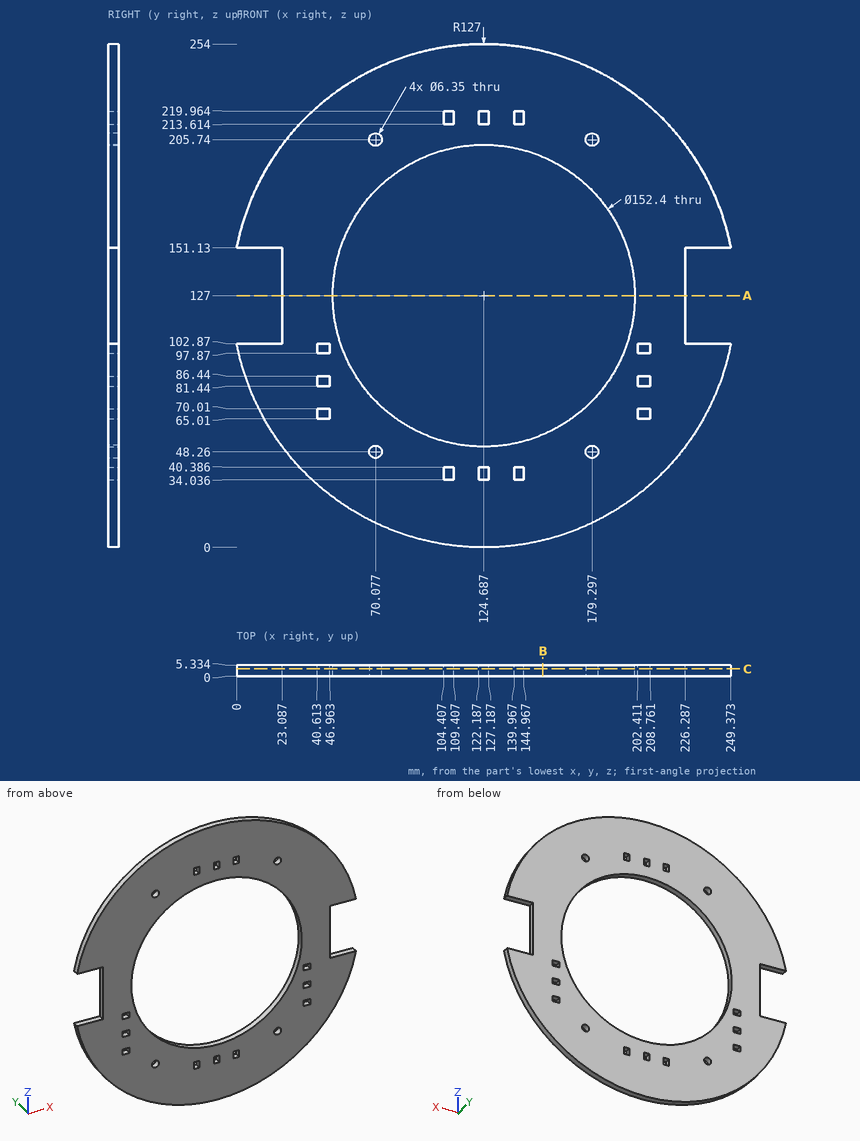
Here's the drawing with two shaded views (mm, measured from the low corner). I have some questions. Give positions to 0.01 mm unless a question says otherwise; leave off trailing zeros. Loops run counter-clockwise (first coordinate to the right, second up) from the corner with the lowest first, then second, coordinate; pieces in that order, holes last. Notation, with made-up numbers: (-24.5, 80.25) - (32.5, 80.25) arc R18 cw to (32.5, 104.25) - close; hole circle Ø6 at (-21.75, 10.25). An arc over 180 degrees is marked (long way). Return JSON: item names as keys, results as strings.
1. I want a section at C-C on y = 3.6. Give the number of separate pieces and of enclosed holes in the cut face, and give its area (3 significant figures).
Output values:
{"separate pieces": "1", "enclosed holes": "17", "area": "29,500 mm²"}
2. I want a section at A-A on z = 127. Please give me the cut outline in (x, y), and give its area (3 significant figures).
Output values:
{"outline": "(23.09, 0) - (48.49, 0) - (48.49, 5.33) - (23.09, 5.33) - close; (200.89, 0) - (226.29, 0) - (226.29, 5.33) - (200.89, 5.33) - close", "area": "271 mm²"}
3. I'm going to push flat-ended pins straight in: pin 1 Ø3 at (y, z) = (2, 136.5) entering from +X; pin 2 Ø1.5 at (y, z) = (3.5, 45.5) entering from -X (1 decimal); pin 3 Ø1.6 at (x, y) = (241, 4) entering from +Z. Where does each tip first touch, or does it pass through?
Output values:
{"pin 1": "stops at x = 226.29", "pin 2": "stops at x = 26.7", "pin 3": "stops at z = 179.78"}
4. I want a section at B-B on x = 154.5. Please give me the cut outline in (y, z) (1 decimal), and give its area (3 significant figures).
Output values:
{"outline": "(0, 3.5) - (5.3, 3.5) - (5.3, 56.9) - (0, 56.9) - close; (0, 197.1) - (5.3, 197.1) - (5.3, 250.5) - (0, 250.5) - close", "area": "569 mm²"}
5. If I drill on line 1 (X direction, y = 0.45, z = 217) (1 decimal); line 2 (Z direction, x = 206.5, y = 3.8) (1 decimal); line 3 (X direction, y = 4.05, z = 205.74), over which ranges is the centre line in solid material (lowest first)?
Output values:
{"line 1": "x = 35.1 to 104.4, 109.4 to 122.2, 127.2 to 140, 145 to 214.3", "line 2": "z = 29.9 to 65, 70 to 81.4, 86.4 to 97.9, 102.9 to 224.1", "line 3": "x = 25.04 to 66.9, 73.25 to 176.12, 182.47 to 224.33"}
